Part model, mm, in its own coordinate system. A direction names the side the tool comes from. Round coordinates to 2 decimals unless told otherwise and drop trailing zeros. Loops run counter-clockwise (first coordinate to the right, second up) from the corner with the lowest first, then second, coordinate; pieces in that order, holes last. Notation, with made-up numbers: (-17, 54.25) -> (-3, 54.25) arc R21 ccw to (-3, 66.25) -> close; hole circle Ø4 at (-28, 38.5). An arc over 180 degrees is marked (long way). Answer as CSV lines item,"result".
from build123d import *

# Parameters (mm, degrees)
F1_DEPTH = 3.175


with BuildPart() as f1:
    # F0 (on Right) → F1 (new body)
    with BuildSketch(Plane.YZ):
        Polygon((-66.040002, 59.831111), (-86.360002, 59.831111), (-86.360002, 52.352222), (-83.185002, 52.352222), (-83.185002, 44.873333), (-86.360002, 44.873333), (-86.360002, 37.394444), (-83.185002, 37.394444), (-83.185002, 29.915556), (-86.360002, 29.915556), (-86.360002, 22.436667), (-83.185002, 22.436667), (-83.185002, 14.957778), (-86.360002, 14.957778), (-86.360002, 7.478889), (-83.185002, 7.478889), (-83.185002, 0), (-86.360002, 0), (-86.360002, -7.478889), (-66.040002, -7.478889), (-66.040002, 0), (-69.215002, 0), (-69.215002, 7.478889), (-66.040002, 7.478889), (-66.040002, 14.957778), (-69.215002, 14.957778), (-69.215002, 22.436667), (-66.040002, 22.436667), (-66.040002, 29.915556), (-69.215002, 29.915556), (-69.215002, 37.394444), (-66.040002, 37.394444), (-66.040002, 44.873333), (-69.215002, 44.873333), (-69.215002, 52.352222), (-66.040002, 52.352222), align=None)
    extrude(amount=F1_DEPTH)


solid = f1.part
Q1. Saw through at B-B, the plane z = 6.5. Write the cut outline in (x, y) (3 decimals).
Geometry results:
outline,"(0, -83.185) -> (3.175, -83.185) -> (3.175, -69.215) -> (0, -69.215) -> close"
Q2. Drop a flat-ended pin along its axis: P1, Ø1, axis at x = 1.5, z = 50.5, coming from the -Y side (3 decimals). Give the stop position or say it passes through.
Geometry results:
P1,"y = -83.185"
Q3. Saw through at A-A, the plane y = -84.5. Write the cut outline in (x, z) (3 decimals), then the cut area to 3 significant figures.
Geometry results:
outline,"(0, -7.479) -> (3.175, -7.479) -> (3.175, 0) -> (0, 0) -> close; (0, 7.479) -> (3.175, 7.479) -> (3.175, 14.958) -> (0, 14.958) -> close; (0, 22.437) -> (3.175, 22.437) -> (3.175, 29.916) -> (0, 29.916) -> close; (0, 37.394) -> (3.175, 37.394) -> (3.175, 44.873) -> (0, 44.873) -> close; (0, 52.352) -> (3.175, 52.352) -> (3.175, 59.831) -> (0, 59.831) -> close"
area,"119 mm2"
Q4. Two-plate mould, pull along Z, no slides. Class faces 1 (the face through (2, -66.04, -4)), 2 (the face through (2, -85, 52.352)), 3 (the face through (2, -85, 29.916)): pulls with the +Z half, pulls with the -Z half, needs draft (parallel to the pull), parting line crosses it, or undercut.
Geometry results:
face 1,"needs draft"
face 2,"undercut"
face 3,"undercut"
Q5. Which spindle directions (+Z, -Z, +X, -X, +Y, -Y) get a long thin tool onto all of the face, cutting with end or side? Do faces 4 (the face through (2, -85, 0)), 5 (the face through (2, -68, 22.437)), 6 (the face through (2, -86.36, -4)). Say none if no direction does.
Geometry results:
face 4,"+X, -X, -Y"
face 5,"+X, -X, +Y"
face 6,"+Z, -Z, +X, -X, -Y"
Q6. Drill centre lines: line 1 along Z through (x, y) = (2.25, -67); line 2 along Y through (x, z) = (1.15, 2) (3 decimals). Where is each one in solid material? Low to high.
Geometry results:
line 1,"-7.48 to 0, 7.48 to 14.96, 22.44 to 29.92, 37.39 to 44.87, 52.35 to 59.83"
line 2,"-83.185 to -69.215"
